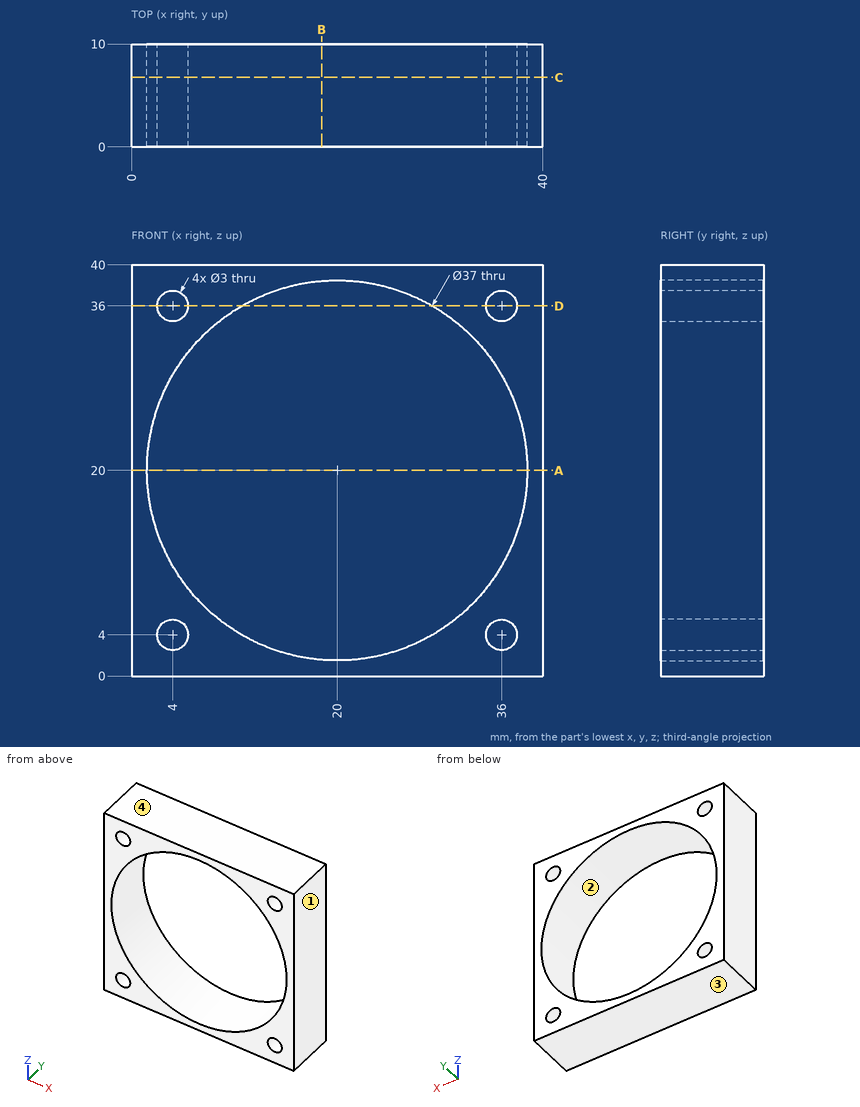
Print and shaded views of the part. All mm, measured from the part's lowest x, y and z. Give positions to 0.01 mm unless a question says otherwise; leave off trailing zeros. Write each loop counter-clockwise with the first axis right and the second up, starting at its lowest first coordinate (ties: lowest second). Pieces come first, ordered by that corner, then holes. Notation, with made-up numbers: (-15.5, 16.25) -> (-6.5, 16.25) arc R33 ccw to (-6.5, 55.25) -> close; hole circle Ø9 at (77, 21). An arc over 180 degrees is marked (long way). Use CSV: the item, a comma, the result in double quotes. Start each with the question number.
1) Cut at A-A on z = 20. List the corners of the cut face in (x, y), plus the area to 3 significant figures.
2) Cut at D-D on z = 36. List the corners of the cut face in (x, y), plus the area to 3 significant figures.
3) Two-plate mould, pull along Z, no slides. Class the marked faces 1, 2, 3 and 4: released by +Z, released by -Z, zero draft, split by the parting line, or undercut.
4) Pin check, flat tip, straight feed: P1, Ø12, axis at x = 19, z = 30, coming from the -Y side. Stop position of the tip, or through.
5) Cut at C-C on y = 6.75. List the corners of the cut face in (x, z), plus the area to 3 significant figures.
6) Cut at B-B on x = 18.5. List the corners of the cut face in (y, z), plus the area to 3 significant figures.
7) Drill centre lines: L1, parallel to X at y = 8.25, z = 4.5; L2, parallel to X at y = 7, z = 36; L3, parallel to Z at x = 37, y = 8.25. Where is each one in solid material? Low to high.
Final values:
1,outline,"(0, 0) -> (1.5, 0) -> (1.5, 10) -> (0, 10) -> close; (38.5, 0) -> (40, 0) -> (40, 10) -> (38.5, 10) -> close"
1,area,"30.0 mm2"
2,outline,"(0, 0) -> (2.5, 0) -> (2.5, 10) -> (0, 10) -> close; (5.5, 0) -> (10.71, 0) -> (10.71, 10) -> (5.5, 10) -> close; (29.29, 0) -> (34.5, 0) -> (34.5, 10) -> (29.29, 10) -> close; (37.5, 0) -> (40, 0) -> (40, 10) -> (37.5, 10) -> close"
2,area,"154 mm2"
3,face 1,"zero draft"
3,face 2,"undercut"
3,face 3,"released by -Z"
3,face 4,"released by +Z"
4,P1,"passes through"
5,outline,"(0, 0) -> (40, 0) -> (40, 40) -> (0, 40) -> close; hole circle Ø37 at (20, 20); hole circle Ø3 at (4, 4); hole circle Ø3 at (4, 36); hole circle Ø3 at (36, 4); hole circle Ø3 at (36, 36)"
5,area,"497 mm2"
6,outline,"(0, 0) -> (10, 0) -> (10, 1.56) -> (0, 1.56) -> close; (0, 38.44) -> (10, 38.44) -> (10, 40) -> (0, 40) -> close"
6,area,"31.2 mm2"
7,L1,"x = 0 to 2.59, 5.41 to 9.9, 30.1 to 34.59, 37.41 to 40"
7,L2,"x = 0 to 2.5, 5.5 to 10.71, 29.29 to 34.5, 37.5 to 40"
7,L3,"z = 0 to 2.88, 5.12 to 12.7, 27.3 to 34.88, 37.12 to 40"
